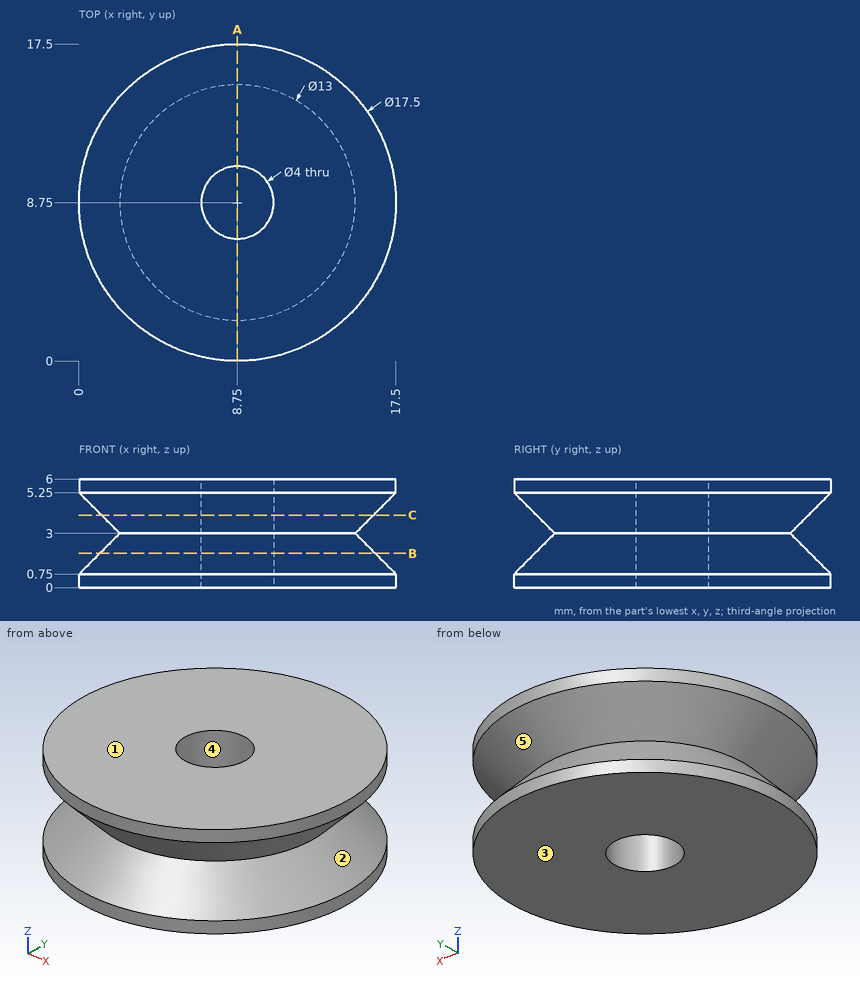
Check sheet for the drawn part. Datum: minimum x, y, z corner. Units: mm. A direction names the side the tool comes from. Coordinates: 2 decimals unless noted, no trailing zeros. Loops run counter-clockwise (first coordinate to the right, second up) from the corner with the lowest first, then second, coordinate; pieces in that order, holes last. Notation, with made-up numbers: (22.25, 68.25) -> (49.25, 68.25) arc R33 cw to (49.25, 106.25) -> close; hole circle Ø8 at (57, 55.25). An arc over 180 degrees is marked (long way). Answer in a Markdown table with one row per item.
1) Depth check by flat-ended pin: P1, Ø2, axis at x = 15.5, z = 2, coming from the +Y side; P2, Ø1.5, axis at x = 13.5, z = 1.5, coming from the -Y side; P3, Ø3, axis at x = 10, z = 3, coming from the -Y side. Enter the tip coordinate at first touch or a pass-through.
The answers:
| item | result |
|---|---|
| P1 | stops at y = 14.32 |
| P2 | stops at y = 1.29 |
| P3 | stops at y = 0.83 |
2) Draft check along X on the marked faces 3, 4 and 5. Enter one of: released by +X, released by -X, zero draft, split by the parting line, or undercut.
The answers:
| item | result |
|---|---|
| face 3 | zero draft |
| face 4 | undercut |
| face 5 | split by the parting line |
3) Access from +Z, -Z, +X, -X, +Y, -Y to the whole of each face (thin tool, end or side, straight path). Record for the marked faces 1 and 2.
The answers:
| item | result |
|---|---|
| face 1 | +Z, +X, -X, +Y, -Y |
| face 2 | none |
4) Section check C-C (z = 4). Record the cut outline in (x, y).
The answers:
| item | result |
|---|---|
| outline | circle Ø15 at (8.75, 8.75); hole circle Ø4 at (8.75, 8.75) |
5) Section check B-B (z = 1.9). Record the cut outline in (x, y).
The answers:
| item | result |
|---|---|
| outline | circle Ø15.2 at (8.75, 8.75); hole circle Ø4 at (8.75, 8.75) |
6) Section check A-A (x = 8.75). Record the cut outline in (y, z), and give its area (3 significant figures).
The answers:
| item | result |
|---|---|
| outline | (0, 0) -> (6.75, 0) -> (6.75, 6) -> (0, 6) -> (0, 5.25) -> (2.25, 3) -> (0, 0.75) -> close; (10.75, 0) -> (17.5, 0) -> (17.5, 0.75) -> (15.25, 3) -> (17.5, 5.25) -> (17.5, 6) -> (10.75, 6) -> close |
| area | 70.9 mm2 |
7) Scan lines: line 1 along Z through (x, y) = (3, 13.5); line 2 along Y through (x, z) = (8, 1.35); line 3 along Y through (x, z) = (8.75, 4.6). Record each from-to range of solid material in increasing order. Write a range as from..to.
The answers:
| item | result |
|---|---|
| line 1 | z = 0..2.04, 3.96..6 |
| line 2 | y = 0.63..6.9, 10.6..16.87 |
| line 3 | y = 0.65..6.75, 10.75..16.85 |
